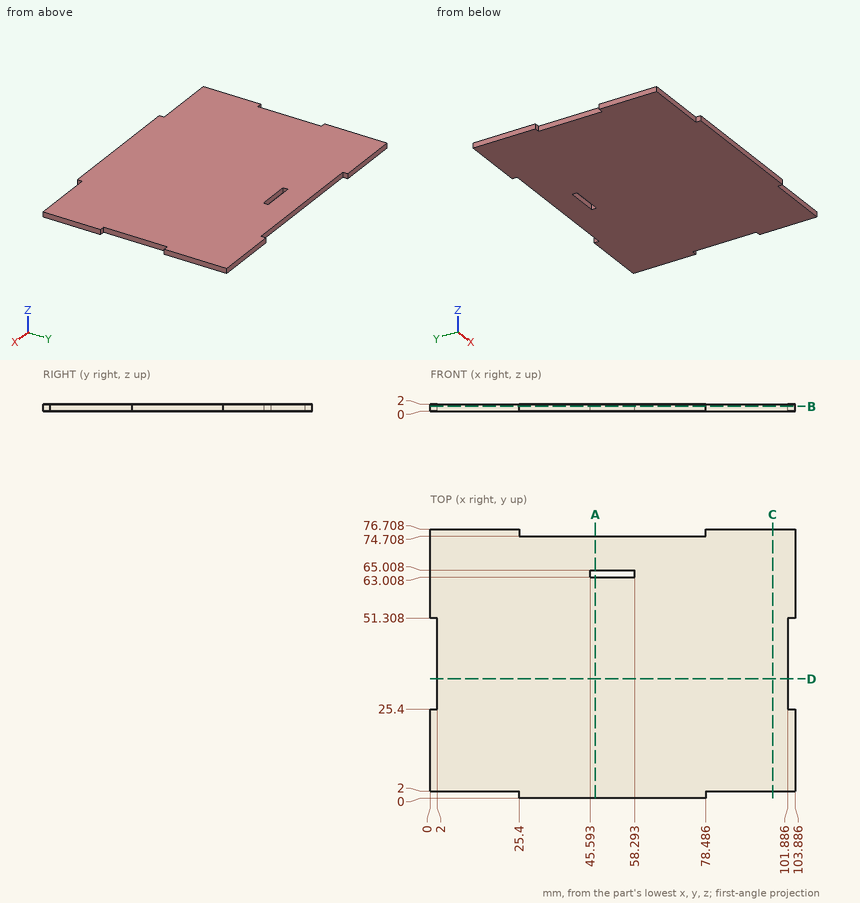
Study the drawing (mm; zero at the part's minimum x, y, z) and answer. Give positions to 0.01 mm unless a question says otherwise; leave off trailing zeros. Write each loop counter-clockwise with the first axis right and the second up, starting at its lowest first coordinate (ties: lowest second). Pieces come first, ordered by that corner, then holes.
Item 1: Find the intervals of material crossed by line 1 along Y through (x, z) = (53.5, 0.4); line 2 along Y through (x, z) = (40.5, 0.2); line 3 along Y through (x, z) = (83, 0.45), in increasing order.
Item 2: Section D-D, the plane y = 34 is taken. Write down the section's boundary in (x, z).
Item 3: Section A-A, the plane x = 47 is taken. Write down the section's boundary in (y, z).
Item 4: Flat-ended cylindrical pins translate along their axes: P1, Ø1, axis at x = 47, z = 1.5, coming from the +Y side; P2, Ø1, axis at y = 37.5, z = 1, coming from the +X side; P3, Ø0.6, axis at x = 103, z = 1.5, coming from the -Y side. Find the tip coordinate at first contact, or state that the pin passes through.
Item 5: Section B-B, the plane z = 1.35 is taken. Write down the section's boundary in (x, y).
Item 6: Section C-C, the plane x = 97.5 is taken. Write down the section's boundary in (y, z).
Completed:
1. line 1: y = 0 to 63.01, 65.01 to 74.71
1. line 2: y = 0 to 74.71
1. line 3: y = 2 to 76.71
2. outline: (2, 0) - (101.89, 0) - (101.89, 2) - (2, 2) - close
3. outline: (0, 0) - (63.01, 0) - (63.01, 2) - (0, 2) - close; (65.01, 0) - (74.71, 0) - (74.71, 2) - (65.01, 2) - close
4. P1: stops at y = 74.71
4. P2: stops at x = 101.89
4. P3: stops at y = 2
5. outline: (0, 2) - (25.4, 2) - (25.4, 0) - (78.49, 0) - (78.49, 2) - (103.89, 2) - (103.89, 25.4) - (101.89, 25.4) - (101.89, 51.31) - (103.89, 51.31) - (103.89, 76.71) - (78.49, 76.71) - (78.49, 74.71) - (25.4, 74.71) - (25.4, 76.71) - (0, 76.71) - (0, 51.31) - (2, 51.31) - (2, 25.4) - (0, 25.4) - close; hole (45.59, 63.01) - (58.29, 63.01) - (58.29, 65.01) - (45.59, 65.01) - close
6. outline: (2, 0) - (76.71, 0) - (76.71, 2) - (2, 2) - close
